from build123d import *

# Parameters (mm, degrees)
SKETCH_1_R      = 1.35
SKETCH_1_W      = 3
SKETCH_1_H      = 6
SKETCH_1_W_2    = 15
SKETCH_1_H_2    = 3
SKETCH_1_W_3    = 22.999
SKETCH_1_H_3    = 12.401
SKETCH_1_W_4    = 2.327
SKETCH_1_H_4    = 1.693
SKETCH_1_W_5    = 2.381
SKETCH_1_H_5    = 1.694
SKETCH_1_W_6    = 10
EXTRUDE_1_DEPTH = 3


with BuildPart() as part:
    # 草图1 → 凸台-拉伸1 (new body)
    with BuildSketch(Plane(origin=(0, 0, 0), x_dir=(-1, 0, 0), z_dir=(0, 0, -1))):
        with BuildLine():
            Line((-28.066816536, 0), (25.933183464, 0))
            ThreePointArc((25.933183464, 0), (28.054503808, 0.878679656), (28.933183464, 3))
            Line((28.933183464, 3), (28.933183464, 41.999))
            ThreePointArc((28.933183464, 41.999), (28.054503808, 44.120320344), (25.933183464, 44.999))
            Line((25.933183464, 44.999), (-28.066816536, 44.999))
            ThreePointArc((-28.066816536, 44.999), (-30.18813688, 44.120320344), (-31.066816536, 41.999))
            Line((-31.066816536, 41.999), (-31.066816536, 3))
            ThreePointArc((-31.066816536, 3), (-30.18813688, 0.878679656), (-28.066816536, 0))
        make_face()
        with Locations(Location((-10.567816536, 42.429, 0), (0, 0, 180))):
            Circle(SKETCH_1_R, mode=Mode.SUBTRACT)
        with Locations(Location((24.432183464, 12.499, 0), (0, 0, 180))):
            Circle(SKETCH_1_R, mode=Mode.SUBTRACT)
        with Locations(Location((-10.567816536, 23.43, 0), (0, 0, 180))):
            Circle(SKETCH_1_R, mode=Mode.SUBTRACT)
        with Locations(Location((-26.567767322, 12.499, 0), (0, 0, 180))):
            Circle(SKETCH_1_R, mode=Mode.SUBTRACT)
        with Locations((-26.566816536, 18.999)):
            Rectangle(SKETCH_1_W, SKETCH_1_H, mode=Mode.SUBTRACT)
        with Locations((-26.566816536, 5.999)):
            Rectangle(SKETCH_1_W, SKETCH_1_H, mode=Mode.SUBTRACT)
        with Locations((-16.067816536, 4.499)):
            Rectangle(SKETCH_1_W_2, SKETCH_1_H_2, mode=Mode.SUBTRACT)
        with Locations((-10.567316536, 32.9995)):
            Rectangle(SKETCH_1_W_3, SKETCH_1_H_3, mode=Mode.SUBTRACT)
        with Locations((18.271683464, 35.4965)):
            Rectangle(SKETCH_1_W_4, SKETCH_1_H_4, mode=Mode.SUBTRACT)
        with Locations((18.298683464, 30.257)):
            Rectangle(SKETCH_1_W_5, SKETCH_1_H_5, mode=Mode.SUBTRACT)
        with Locations((24.433183464, 18.999)):
            Rectangle(SKETCH_1_W, SKETCH_1_H, mode=Mode.SUBTRACT)
        with Locations((24.433183464, 5.999)):
            Rectangle(SKETCH_1_W, SKETCH_1_H, mode=Mode.SUBTRACT)
        with Locations((16.432183464, 4.499)):
            Rectangle(SKETCH_1_W_6, SKETCH_1_H_2, mode=Mode.SUBTRACT)
    extrude(amount=-EXTRUDE_1_DEPTH)


solid = part.part
Design review of the part built by this model. Coordinates are the model's own, in mm. A direction names the side the tool comes from. Round coordinates to 2 decimals unless told otherwise and drop trailing zeros. Order: outer loops, then holes, each group sorted by start corner. A loop starts at its lowest first (then second) coordinate and runs counter-clockwise, first axis right, second up. Notation, with made-up numbers: M 32,36 L 50,36 A23 cw 50,58 Z; hole C -6,8 d5. An arc over 180 degrees is marked long. Answer as CSV lines item,"result". Start each with the question number.
1) The part is to be moulded in two halves that separate along X. For faces 3 (the face through (1, 23, 3)), 4 (the face through (-0.932, 33, 1)), 5 (the face through (31.067, 23, 1)), 6 (the face through (8.568, 4, 1)), say which applies: +X half, -X half, draft (parallel to the pull), parting line (faces both ways), or undercut.
2) Add section A-A (y = 23.43). Give the boundary of the cut face in (x, z).
3) Wall thickness on line 1 along Y through (x, z) = (18.5, 2.5); line 2 along X through (y, z) = (5, 1.85); line 3 along X through (y, z) = (30, 2.2): over which ranges is each line inside the solid? List them lowest first. Write a range as [from, to].
4) Add section B-B (y = 38.5). Give the boundary of the cut face in (x, z), then the cut area to 3 significant figures.
5) Tool access review of faces 1 (the face through (11, 26.799, 1)), 2 (the face through (1, 44.999, 1)): name each direction out of +Z, -Z, +X, -X, +Y, -Y from which nothing blocks a thin tool from reaching the whole face with its end or side.
6) Add section C-C (z = 1.25). Give the number of separate pieces and of enclosed holes in the cut face, then the cut area to 3 significant figures.
Resolved:
1,face 3,"draft"
1,face 4,"undercut"
1,face 5,"+X half"
1,face 6,"undercut"
2,outline,"M -28.93,0 L 9.22,0 L 9.22,3 L -28.93,3 Z; M 11.92,0 L 31.07,0 L 31.07,3 L 11.92,3 Z"
3,line 1,"[0, 3], [6, 26.8], [39.2, 45]"
3,line 2,"[-28.93, -25.93], [-22.93, -21.43], [-11.43, 8.57], [23.57, 25.07], [28.07, 31.07]"
3,line 3,"[-28.93, -19.49], [-17.11, -0.93], [22.07, 31.07]"
4,outline,"M -28.93,0 L -0.93,0 L -0.93,3 L -28.93,3 Z; M 22.07,0 L 31.07,0 L 31.07,3 L 22.07,3 Z"
4,area,"111 mm^2"
5,face 1,"+Z, -Z"
5,face 2,"+Z, -Z, +X, -X, +Y"
6,separate pieces,"1"
6,enclosed holes,"13"
6,area,"2,230 mm^2"
